Source: CAD feature listing. Evaluate the final solid. Frame: model axes, mm. Face numbers are marked on the shaded views. A direction names the side the tool comes from. Coordinates: 2 decimals unless noted, no trailing zeros. Order: outer loops, then holes, each group sorted by start corner. A loop starts at its lowest first (then second) coordinate and runs counter-clockwise, first axis right, second up.
```python
from build123d import *

# Parameters (mm, degrees)
CROQUIS1_W              = 67
CROQUIS1_H              = 22
CROQUIS1_W_2            = 21
CROQUIS1_H_2            = 21
SALIENTE_EXTRUIR1_DEPTH = 32
CROQUIS1_2_W            = 21
CROQUIS1_2_H            = 21
SALIENTE_EXTRUIR2_DEPTH = 4
CORTAR_EXTRUIR1_DEPTH   = 52.285962992


with BuildPart() as part:
    # Croquis1 → Saliente-Extruir1 (new body)
    with BuildSketch(Plane(origin=(0, 0, 0), x_dir=(1, 0, 0), z_dir=(0, 1, 0))):
        Rectangle(CROQUIS1_W, CROQUIS1_H)
        Rectangle(CROQUIS1_W_2, CROQUIS1_H_2, mode=Mode.SUBTRACT)
        with Locations((-22, 0)):
            Rectangle(CROQUIS1_W_2, CROQUIS1_H_2, mode=Mode.SUBTRACT)
        with Locations((22, 0)):
            Rectangle(CROQUIS1_W_2, CROQUIS1_H_2, mode=Mode.SUBTRACT)
    extrude(amount=SALIENTE_EXTRUIR1_DEPTH)

    # Croquis1<2> → Saliente-Extruir2 (add)
    with BuildSketch(Plane(origin=(0, 0, 0), x_dir=(1, 0, 0), z_dir=(0, 1, 0))):
        Rectangle(CROQUIS1_2_W, CROQUIS1_2_H)
        with Locations((-22, 0)):
            Rectangle(CROQUIS1_2_W, CROQUIS1_2_H)
        with Locations((22, 0)):
            Rectangle(CROQUIS1_2_W, CROQUIS1_2_H)
    extrude(amount=SALIENTE_EXTRUIR2_DEPTH)

    # Croquis2 → Cortar-Extruir1 (cut, through all)
    with BuildSketch(Plane.XY.offset(11)):
        with BuildLine():
            Line((-25, 32), (-25, 9))
            ThreePointArc((-25, 9), (-22, 6), (-19, 9))
            Line((-19, 9), (-19, 32))
            Line((-19, 32), (-25, 32))
        make_face()
        with BuildLine():
            Line((-3, 32), (-3, 9))
            ThreePointArc((-3, 9), (0, 6), (3, 9))
            Line((3, 9), (3, 32))
            Line((3, 32), (-3, 32))
        make_face()
        with BuildLine():
            Line((19, 32), (19, 9))
            ThreePointArc((19, 9), (22, 6), (25, 9))
            Line((25, 9), (25, 32))
            Line((25, 32), (19, 32))
        make_face()
    extrude(amount=-CORTAR_EXTRUIR1_DEPTH, mode=Mode.SUBTRACT)


solid = part.part
```
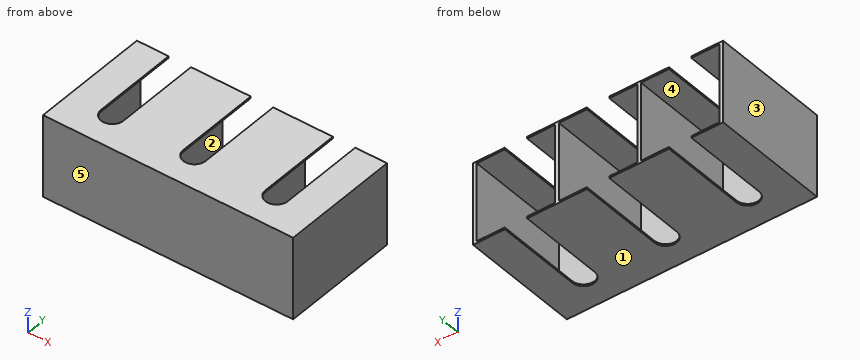
1. Material intervals for line 1 along X through (y, z) = (25.5, -5.25); line 2 along Z through (x, y) = (19, 8); line 3 along Y through (x, z) = (10, -8), sorted ascending.
2. Section query B-B, the plane z = 7. Output: boundary loops of the cut face in (x, y).
3. Section query C-C, the plane y = 11.5. Count the separate pieces of the cut face and the enclosed holes in it, plus the area to 3 significant figures.
4. Contact query for a flat-ended pin moving along its axis: P1, Ø6.5, axis at x = -26, z = 4.5, coming from the +Y side. Output: stop coordinate, or through.
5. Section query D-D, the plane x = 0. Output: boundary loops of the cut face in (y, z), plus the area to 3 significant figures.
6. Section query A-A, the plane x = 9. Output: boundary loops of the cut face in (y, z), plus the area to 3 significant figures.
7. Draft query along X for the marked faces 1, 2 and 3. Return one class per face: +X half, -X half, draft (parallel to the pull), parting line (faces both ways), or undercut.
8. Access query for the marked faces 4 and 5. Directions: +Z, -Z, +X, -X, +Y, -Y. A direction counts if a zero-diameter tool reaches every point of the face in a straight line with its end or side. Return the directions, or none.
Answer key:
1. line 1: x = -33.5 to -32.5, -11.5 to -10.5, 10.5 to 11.5, 32.5 to 33.5
1. line 2: z = -11 to -10.5, 10.5 to 11
1. line 3: y = 0 to 4
2. outline: (-33.5, 0) - (33.5, 0) - (33.5, 32) - (32.5, 32) - (32.5, 4) - (11.5, 4) - (11.5, 32) - (10.5, 32) - (10.5, 4) - (-10.5, 4) - (-10.5, 32) - (-11.5, 32) - (-11.5, 4) - (-32.5, 4) - (-32.5, 32) - (-33.5, 32) - close
3. separate pieces: 4
3. enclosed holes: 0
3. area: 133 mm2
4. P1: stops at y = 4
5. outline: (0, -11) - (6, -11) - (6, -10.5) - (4, -10.5) - (4, 10.5) - (6, 10.5) - (6, 11) - (0, 11) - close
5. area: 90.0 mm2
6. outline: (0, -11) - (32, -11) - (32, -10.5) - (4, -10.5) - (4, 10.5) - (32, 10.5) - (32, 11) - (0, 11) - close
6. area: 116 mm2
7. face 1: draft
7. face 2: undercut
7. face 3: -X half
8. face 4: +Y
8. face 5: +Z, -Z, +X, -X, -Y
